```python
from build123d import *

# Parameters (mm, degrees)
F0_W     = 120
F0_H     = 90
F1_DEPTH = 5
F3_DEPTH = 5
F4_R     = 30
F5_DEPTH = 5
F6_R     = 3
F7_DEPTH = 5


with BuildPart() as f1:
    # F0 (on Front) → F1 (new body)
    with BuildSketch(Plane.XZ):
        Rectangle(F0_W, F0_H)
    extrude(amount=F1_DEPTH)

    # F2 (on face) → F3 (join)
    with BuildSketch(Plane.XZ.offset(5)):
        with BuildLine():
            Line((-45, 40), (-55, 18))
            Line((-55, 18), (-55, -18))
            Line((-55, -18), (-52, -18))
            ThreePointArc((-52, -18), (-40.125791, -21.574479), (-35, -32.866069))
            Line((-35, -32.866069), (-35, -40))
            Line((-35, -40), (35, -40))
            Line((35, -40), (35, -32.866069))
            ThreePointArc((35, -32.866069), (40.125791, -21.574479), (52, -18))
            Line((52, -18), (55, -18))
            Line((55, -18), (55, 25))
            ThreePointArc((55, 25), (50.606602, 35.606602), (40, 40))
            Line((40, 40), (-45, 40))
        make_face()
    extrude(amount=F3_DEPTH)

    # F4 (on face) → F5 (cut)
    with BuildSketch(Plane.XZ.offset(10)):
        Circle(F4_R)
    extrude(amount=-F5_DEPTH, mode=Mode.SUBTRACT)

    # F6 (on face) → F7 (cut)
    with BuildSketch(Plane.XZ.offset(5)):
        with Locations((-14.14, 14.144271)):
            Circle(F6_R)
        with Locations((0, 20)):
            Circle(F6_R)
        with Locations((14.14, 14.144271)):
            Circle(F6_R)
        with Locations((20, 0)):
            Circle(F6_R)
        with Locations((14.144271, -14.14)):
            Circle(F6_R)
        with Locations((0, -20)):
            Circle(F6_R)
        with Locations((-14.144271, -14.14)):
            Circle(F6_R)
        with Locations((-20, 0)):
            Circle(F6_R)
    extrude(amount=-F7_DEPTH, mode=Mode.SUBTRACT)


solid = f1.part
```
Source: CAD feature listing. Evaluate the final solid. Frame: model axes, mm. A direction names the side the tool comes from. Give positions to 0.01 mm unless a question says otherwise; leave off trailing zeros. Loops run counter-clockwise (first coordinate to the right, second up) from the corner with the lowest first, then second, coordinate; pieces in that order, holes last. Notation, with made-up numbers: (6.5, 24.5) - (41.5, 24.5) arc R29 cw to (41.5, 45.5) - close; hole circle Ø1 at (81, 30). An arc over 180 degrees is marked (long way). Use CSV: the item, a comma, the result in double quotes. Start each with the question number.
1. Draft query along Z for faces 1 (the cylindrical face through (-40.26, -7.46, -21.46)), 2 (the flat face through (-2, -7, 40)), 3 (the cylindrical face through (-0.65, -2.54, -22.93)). Return one class per face: +Z half, -Z half, draft (parallel to the pull), parting line (faces both ways), or undercut.
2. Section C-C (z = 0). Output: boundary loops of the cut face in (x, y).
3. Section A-A (x = 0). Output: boundary loops of the cut face in (y, z).
4. Section B-B (y = -8.25). Output: boundary loops of the cut face in (x, z).
5. Ray query, L1, parallel to Z at x = 14.14, y = -1; L2, parallel to Z at x = 20, y = -2.4; L3, parallel to X at y = -3.5, z = 12.5. Return the intervals inside material, ascending.
6. Reachability of faces 4 (the flat face through (53, -7, -18)), 5 (the flat face through (-55, -7, 0)), 6 (the flat face through (-54, -7, -18)) from +Z, -Z, +X, -X, +Y, -Y: full face, straight path, thin tool, end or side. Return the list, or none.
7. Section D-D (x = -50). Output: boundary loops of the cut face in (y, z), then the cut area to 3 significant figures.
8. Pin query (flat end, axial travel): pin 1 (2.5 mm diameter, centred on x = 4, y = -8, fed in from -Z); pin 2 (1 mm diameter, centred on x = 4, z = 12, fed in from -Y); pin 3 (2.5 mm diameter, centred on y = -8, z = 7, fed in from -X). Return the tip coordinate at first contact, or that it passes through.
Response:
1,face 1,"-Z half"
1,face 2,"+Z half"
1,face 3,"undercut"
2,outline,"(-60, -5) - (-55, -5) - (-55, -10) - (-30, -10) - (-30, -5) - (-23, -5) - (-23, 0) - (-60, 0) - close; (-17, -5) - (17, -5) - (17, 0) - (-17, 0) - close; (23, -5) - (30, -5) - (30, -10) - (55, -10) - (55, -5) - (60, -5) - (60, 0) - (23, 0) - close"
3,outline,"(-10, -40) - (-5, -40) - (-5, -45) - (0, -45) - (0, -23) - (-5, -23) - (-5, -30) - (-10, -30) - close; (-10, 30) - (-5, 30) - (-5, 23) - (0, 23) - (0, 45) - (-5, 45) - (-5, 40) - (-10, 40) - close; (-5, -17) - (0, -17) - (0, 17) - (-5, 17) - close"
4,outline,"(-55, -18) - (-52, -18) arc R15 cw to (-35, -32.87) - (-35, -40) - (35, -40) - (35, -32.87) arc R15 cw to (52, -18) - (55, -18) - (55, 25) arc R15 ccw to (40, 40) - (-45, 40) - (-55, 18) - close; hole circle Ø60 at (0, 0)"
5,L1,"-45 to -17.14, -11.14 to 11.14, 17.14 to 45"
5,L2,"-45 to -3, 3 to 45"
5,L3,"-60 to -16.65, -11.63 to 11.63, 16.65 to 60"
6,face 4,"-Z, +X, -Y"
6,face 5,"+Z, -Z, -X, -Y"
6,face 6,"-Z, -X, -Y"
7,outline,"(-10, -17.87) - (-5, -17.87) - (-5, -45) - (0, -45) - (0, 45) - (-5, 45) - (-5, 29) - (-10, 29) - close"
7,area,"684 mm²"
8,pin 1,"z = -40"
8,pin 2,"y = -5"
8,pin 3,"x = -55"
